from build123d import *

# Parameters (mm, degrees)
F0_R     = 20.6375062807
F0_R_2   = 2.15265
F0_R_3   = 12.7000062807
F1_DEPTH = 8.001
F3_DEPTH = 8.001
F4_COUNT = 4
F4_ANGLE = 270
F5_R     = 0.762


with BuildPart() as f1:
    # F0 (on Top) → F1 (new body)
    with BuildSketch(Plane.XY):
        Circle(F0_R)
        with Locations((-11.7865906, -11.7865906)):
            Circle(F0_R_2, mode=Mode.SUBTRACT)
        with Locations((11.7865906, -11.7865906)):
            Circle(F0_R_2, mode=Mode.SUBTRACT)
        with Locations((-11.7865906, 11.7865906)):
            Circle(F0_R_2, mode=Mode.SUBTRACT)
        Circle(F0_R_3, mode=Mode.SUBTRACT)
        with Locations((11.7865906, 11.7865906)):
            Circle(F0_R_2, mode=Mode.SUBTRACT)
    extrude(amount=F1_DEPTH)

    # F2 (on face) → F3 (cut, through all)
    with BuildSketch(Plane(origin=(0, 0, 0), x_dir=(1, 0, 0), z_dir=(0, 0, -1))):
        with BuildLine():
            ThreePointArc((10.8660418044, -15.6471043582), (8.7251193967, -14.3121342314), (7.8214782953, -11.9564757766))
            ThreePointArc((7.8214782953, -11.9564757766), (0, -14.2875062807), (-7.8214782953, -11.9564757766))
            ThreePointArc((-7.8214782953, -11.9564757766), (-8.7251193967, -14.3121342314), (-10.8660418044, -15.6471043582))
            ThreePointArc((-10.8660418044, -15.6471043582), (0, -19.0500062807), (10.8660418044, -15.6471043582))
        make_face()
    f3 = extrude(amount=-F3_DEPTH, mode=Mode.SUBTRACT)

    # F4: F3 ×4 about axis
    f4_axis = Axis((0, 0, 0), (0, 0, -1))
    for i in range(1, F4_COUNT):
        add(f3.rotate(f4_axis, i * F4_ANGLE / (F4_COUNT - 1)), mode=Mode.SUBTRACT)

    # F5
    f5_edges = [f1.edges().sort_by_distance(p)[0] for p in [
        (-7.821478, 11.956476, 4.0005),
        (7.821478, 11.956476, 4.0005),
        (-11.956476, -7.821478, 4.0005),
        (-11.956476, 7.821478, 4.0005),
        (-7.821478, -11.956476, 4.0005),
        (7.821478, -11.956476, 4.0005),
        (11.956476, 7.821478, 4.0005),
        (11.956476, -7.821478, 4.0005),
    ]]
    fillet(f5_edges, radius=F5_R)


solid = f1.part
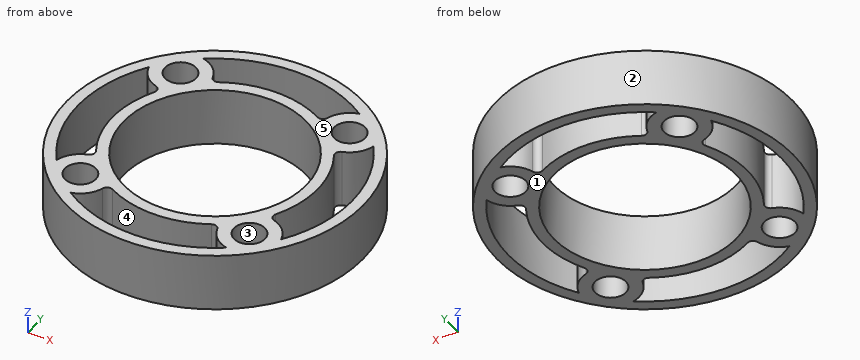
Geometry: final body of the model. Coordinates: model frame, mm. Face numbers are marked on the shaded views. A direction names the side the tool comes from. Round coordinates to 2 decimals unless told otherwise and drop trailing zeros. Loops run counter-clockwise (first coordinate to the right, second up) from the corner with the lowest first, then second, coordinate; pieces in that order, holes last. Notation, with made-up numbers: (73.5, 55.5) -> (86.5, 55.5) arc R22 ccw to (86.5, 76.5) -> close; hole circle Ø3 at (35, 13). An arc over 180 degrees is marked (long way). One line per question, with ' | ' between items. Start each with the question number.
1. Section D-D on z = 6. Count the separate pieces of the cut face and the enclosed holes in it, and give its area (3 significant figures).
2. Set-up query: the marked faces 4 and 5. Return all of +Z, -Z, +X, -X, +Y, -Y with unobstructed straight access to the full face (end or side cutting, diameter ignored); none if empty.
3. Line query: line 1 along Y through (x, z) = (-2.5, 4.25); line 2 along Y through (x, z) = (7.5, 2.75); line 3 along X through (y, z) = (7, 5.75). Output: solid intervals per line, ascending. Write a range as [from, to].
4. Section C-C on x = -15. Output: boundary loops of the cut face in (y, z), and give its area (3 significant figures).
5. Contact query for flat-ended pins moving along their axis: pin 1 (1 mm diameter, centred on y = 14.5, z = 4, fed in from -X); pin 2 (2 mm diameter, centred on y = 6.5, z = 6.5, fed in from +X); pin 3 (1.5 mm diameter, centred on y = 12.5, z = 1.5, fed in from -X). Output: stop coordinate, or through.
6. Section A-A on y = 0. Output: boundary loops of the cut face in (x, z), and give its area (3 significant figures).
7. Mould query, pull axis X, two halves, no side actions, for the marked faces 1, 2 and 3. Classes: pulls with the +X half, pulls with the -X half, needs draft (parallel to the pull), parting line crosses it, or undercut.
Returned:
1) separate pieces: 1 | enclosed holes: 9 | area: 418 mm2
2) face 4: +Z, -Z | face 5: +Z, +X, -X, +Y, -Y
3) line 1: y = [-20.49, -18.89], [-14.07, -12.45], [12.45, 14.07], [18.89, 20.49] | line 2: y = [-19.23, -17.51], [-12.45, -10.25], [10.25, 12.45], [17.51, 19.23] | line 3: x = [-19.41, -17.72], [-12.47, -10.6], [10.6, 12.47], [17.72, 19.41]
4) outline: (-14.17, 0) -> (-9.46, 0) -> (-9.46, 8) -> (-14.17, 8) -> close; (9.46, 0) -> (14.17, 0) -> (14.17, 8) -> (9.46, 8) -> close | area: 75.5 mm2
5) pin 1: stops at x = -15.16 | pin 2: stops at x = 19.89 | pin 3: stops at x = -16.97
6) outline: (-20.64, 0) -> (-19.05, 0) -> (-19.05, 8) -> (-20.64, 8) -> close; (-14.29, 0) -> (-12.7, 0) -> (-12.7, 8) -> (-14.29, 8) -> close; (12.7, 0) -> (14.29, 0) -> (14.29, 8) -> (12.7, 8) -> close; (19.05, 0) -> (20.64, 0) -> (20.64, 8) -> (19.05, 8) -> close | area: 50.8 mm2
7) face 1: needs draft | face 2: parting line crosses it | face 3: undercut
